Drawing for the job (mm, zero at the part's lowest x, y, z). Give positions to 0.01 mm unless a question says otherwise; leave off trailing zeros. Write each loop counter-clockwise with the first axis right and the second up, starting at its lowest first coordinate (ties: lowest second). Pieces come first, ordered by that corner, then holes. Notation, with made-up numbers: M -3,36.25 L 3,36.25 A30 cw 3,62.25 Z; hole C 10.5,70 d11. An arc over 180 degrees is marked long. Answer as a JSON object with one key per item and string values. Group by question number.
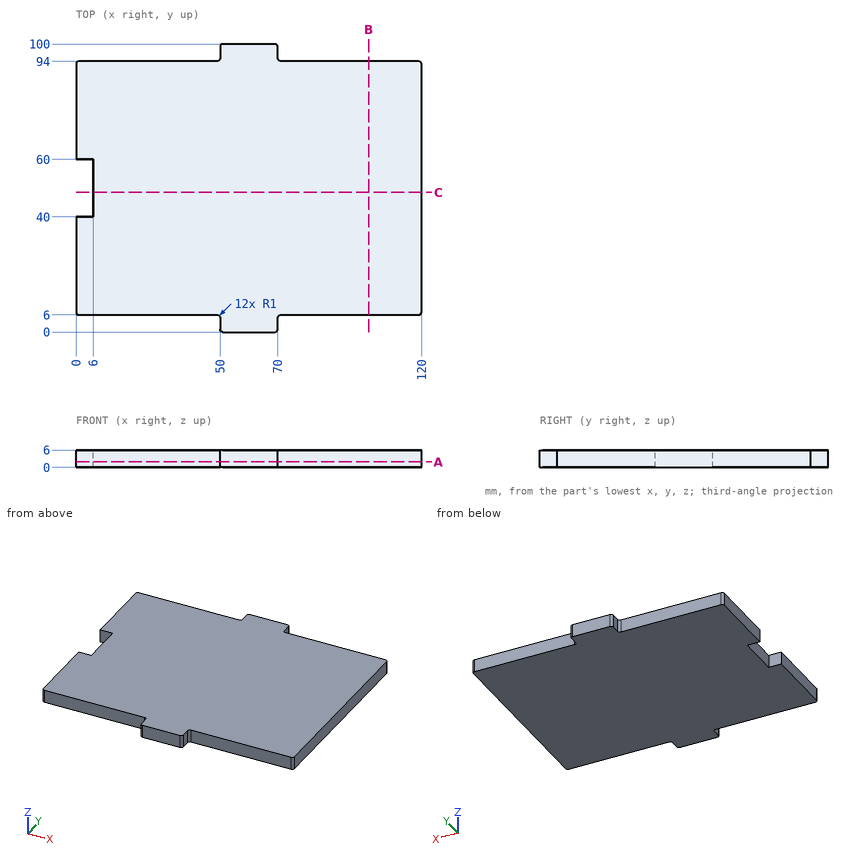
Q1. Slice it at B-B, the plane x = 101.5. Write the cut outline in (y, z).
Q2. Wall check: L1, parallel to Y at x = 16.5, z = 4.65; L2, parallel to X at y = 41.5, z = 3; L3, parallel to X at y = 93.5, z = 5. Give the ranges that are in metal, low to high.
Q3. Slice it at A-A, the plane z = 1.9. Write the cut outline in (x, y).
Q4. Slice it at C-C, the plane y = 48.5. Write the cut outline in (x, z).
Q5. Drop flat-ended pins along their axis: P1, Ø1.8, axis at x = 3.5, z = 3, coming from the +Y side; P2, Ø2, axis at y = 97, z = 2, coming from the -X side; P3, Ø3, axis at x = 19.5, z = 1.5, coming from the -Y side. Give the stop position or say it passes through.
Solved:
{
 "1": {"outline": "M 6,0 L 94,0 L 94,6 L 6,6 Z"},
 "2": {"L1": "y = 6 to 94", "L2": "x = 6 to 120", "L3": "x = 0.13 to 119.87"},
 "3": {"outline": "M 0,7 A1 ccw 1,6 L 49,6 A1 cw 50,5 L 50,1 A1 ccw 51,0 L 69,0 A1 ccw 70,1 L 70,5 A1 cw 71,6 L 119,6 A1 ccw 120,7 L 120,93 A1 ccw 119,94 L 71,94 A1 cw 70,95 L 70,99 A1 ccw 69,100 L 51,100 A1 ccw 50,99 L 50,95 A1 cw 49,94 L 1,94 A1 ccw 0,93 L 0,60 L 6,60 L 6,40 L 0,40 Z"},
 "4": {"outline": "M 6,0 L 120,0 L 120,6 L 6,6 Z"},
 "5": {"P1": "stops at y = 94", "P2": "stops at x = 50", "P3": "stops at y = 6"}
}
